Geometry: final body of the model. Coordinates: model frame, mm. A direction names the side the tool comes from. Give positions to 0.01 mm unless a question says otherwise; leave off trailing zeros. Write each loop counter-clockwise with the first axis right and the second up, starting at its lowest first coordinate (ties: lowest second). Pieces come first, ordered by that corner, then holes. Notation, with made-up numbers: (-5, 87) - (7, 87) arc R19 ccw to (7, 108) - close; hole circle Ø1 at (-20.75, -19). An arc over 180 degrees is marked (long way). One line per question, with ' | ' between items. Start each with the question number.
```python
from build123d import *

# Parameters (mm, degrees)
SKETCH_1_W               = 75
SKETCH_1_H               = 75
EXTRUDE_1_DEPTH          = 5.5
FILLET_1_R               = 5
SKETCH_2_R               = 3.5
CUT_EXTRUDE_1_DEPTH      = 54.31744555
PATTERN_CIRCULAR_1_COUNT = 4
SKETCH_3_R               = 10
CUT_EXTRUDE_2_DEPTH      = 3
SKETCH_4_R               = 35
EXTRUDE_2_DEPTH          = 7
SKETCH_5_R               = 30
EXTRUDE_3_DEPTH          = 55
SKETCH_6_W               = 50
SKETCH_6_H               = 55
EXTRUDE_4_DEPTH          = 26.5
FILLET_2_R               = 15
SKETCH_7_W               = 38
SKETCH_7_H               = 30
CUT_EXTRUDE_3_DEPTH      = 114.606777967
SKETCH_9_R               = 25
EXTRUDE_5_DEPTH          = 12.5
EXTRUDE_6_REACH          = 118.916
SKETCH_8_R               = 2.5
FILLET_3_R               = 15


with BuildPart() as part:
    # Sketch 1 → Extrude 1 (new body)
    with BuildSketch(Plane.XY):
        Rectangle(SKETCH_1_W, SKETCH_1_H)
    extrude(amount=EXTRUDE_1_DEPTH)

    # Fillet 1
    fillet_1_edges = [part.edges().sort_by_distance(p)[0] for p in [
        (-37.5, 37.5, 2.75),
        (37.5, 37.5, 2.75),
        (37.5, -37.5, 2.75),
        (-37.5, -37.5, 2.75),
    ]]
    fillet(fillet_1_edges, radius=FILLET_1_R)

    # Sketch 2 → Cut-Extrude 1 (cut, through all)
    with BuildSketch(Plane.XY.offset(5.5)):
        with Locations((-29, 29)):
            Circle(SKETCH_2_R)
    cut_extrude_1 = extrude(amount=-CUT_EXTRUDE_1_DEPTH, mode=Mode.SUBTRACT)

    # Pattern Circular 1: Cut-Extrude 1 ×4 about axis
    pattern_circular_1_axis = Axis((0, 0, 0), (0, 0, 1))
    for i in range(1, PATTERN_CIRCULAR_1_COUNT):
        add(cut_extrude_1.rotate(pattern_circular_1_axis, i * 360 / PATTERN_CIRCULAR_1_COUNT), mode=Mode.SUBTRACT)

    # Sketch 3 → Cut-Extrude 2 (cut)
    with BuildSketch(Plane.XY.offset(5.5)):
        Circle(SKETCH_3_R)
    extrude(amount=-CUT_EXTRUDE_2_DEPTH, mode=Mode.SUBTRACT)

    # Sketch 4 → Extrude 2 (add)
    with BuildSketch(Plane(origin=(0, 0, 0), x_dir=(-1, 0, 0), z_dir=(0, 0, -1))):
        with Locations(Location((0, 0, 0), (0, 0, 180))):
            Circle(SKETCH_4_R)
    extrude(amount=EXTRUDE_2_DEPTH)

    # Sketch 5 → Extrude 3 (add)
    with BuildSketch(Plane(origin=(0, 0, -7), x_dir=(-1, 0, 0), z_dir=(0, 0, -1))):
        Circle(SKETCH_5_R)
    extrude(amount=EXTRUDE_3_DEPTH)

    # Sketch 6 → Extrude 4 (add, symmetric)
    with BuildSketch(Plane(origin=(0, 0, 0), x_dir=(1, 0, 0), z_dir=(0, 1, 0))):
        with Locations((25, 34.5)):
            Rectangle(SKETCH_6_W, SKETCH_6_H)
    extrude(amount=EXTRUDE_4_DEPTH, both=True)

    # Fillet 2
    fillet_2_edges = [part.edges().sort_by_distance(p)[0] for p in [
        (50, 0, -7),
    ]]
    fillet(fillet_2_edges, radius=FILLET_2_R - 0.0001)  # a hair under: the kernel refuses the full size

    # Sketch 7 → Cut-Extrude 3 (cut, through all)
    with BuildSketch(Plane(origin=(50, 0, 0), x_dir=(0, 0, -1), z_dir=(1, 0, 0))):
        with Locations((43, 0)):
            Rectangle(SKETCH_7_W, SKETCH_7_H)
    extrude(amount=-CUT_EXTRUDE_3_DEPTH, mode=Mode.SUBTRACT)

    # Extrude 6: up to this face of the body (flat: up to its plane)
    extrude_6_end = Plane(part.part.faces().sort_by_distance((31.665133936, -26.5, -35.104709871))[0])
    # Sketch 8 → Extrude 6 (add, up to the picked face)
    with BuildSketch(Plane(origin=(0, 26.5, 0), x_dir=(1, 0, 0), z_dir=(0, 1, 0)), mode=Mode.PRIVATE) as extrude_6_sk1:
        with Locations(Location((36, 51.5, 0), (0, 0, 270))):
            Circle(SKETCH_8_R)
    extrude_6_tool1 = split(extrude(extrude_6_sk1.sketch, amount=-EXTRUDE_6_REACH, mode=Mode.PRIVATE), bisect_by=extrude_6_end, keep=Keep.BOTH, mode=Mode.PRIVATE)


with BuildPart() as body_2:
    # Sketch 9 → Extrude 5 (new, symmetric)
    with BuildSketch(Plane(origin=(0, 0, 0), x_dir=(1, 0, 0), z_dir=(0, 1, 0))):
        with Locations(Location((36, 51.5, 0), (0, 0, 270))):
            Circle(SKETCH_9_R)
    extrude(amount=EXTRUDE_5_DEPTH, both=True)


with BuildPart() as part_1:
    add(part.part)

    add(body_2.part)  # Extrude 6 merges body 2
    add(extrude_6_tool1.solids().sort_by(Axis((36, 26.5, -51.5), (0, -1, 0)))[0])

    # Fillet 3
    fillet_3_edges = [part_1.edges().sort_by_distance(p)[0] for p in [
        (50, 20.75, -62),
        (50, -20.75, -62),
    ]]
    fillet(fillet_3_edges, radius=FILLET_3_R)


solid = part_1.part
```
1) Section D-D, the plane x = 29. Output: boundary loops of the cut face in (y, z).
2) First-contact query: pin 1 Ø1.5 at (y, z) = (-12.5, -8.5) entering from +X; pin 2 Ø20 at (y, z) = (5.5, -30) entering from +X; pin 3 Ø4 at (y, z) = (-17, -4.5) entering from +X; pin 4 Ø11 at (x, y) = (-29, -29) entering from +Z. Flat tips, straight axial feed; report the tip coordinate or a pass-through.
3) Pull-direction query (Y, two-part tool) for faces 6 (the cylindrical face through (-36.07, -36, 2.79)), 7 (the cylindrical face through (-32.47, -29.46, 2.79)), 8 (the flat face through (-37.5, 0, 3)), 9 (the flat face through (0, 0, 2.5)); classes: +Y half, -Y half, draft (parallel to the pull), parting line (faces both ways), or undercut.
4) Reachability of faces 1 (the flat face through (37.5, 0, 3)), 2 (the cylindrical face through (45.72, -20.83, -57.49)), 3 (the cylindrical face through (27.12, -31.95, 2.79)), 4 (the cylindrical face through (45.72, 20.67, -57.49)), 5 (the flat face through (-31, 17, 0)) from +Z, -Z, +X, -X, +Y, -Y: full face, straight path, thin tool, end or side. Return the list, or none.
5) Section B-B, the plane x = 45. Output: boundary loops of the cut face in (y, z).
6) Line query: L1, parallel to X at y = -29, z = 1.3; L2, parallel to Y at x = 49, z = -35.5. Output: solid intervals per line, ascending.
7) Section C-C, the plane z = -51.5. Output: boundary loops of the cut face in (x, y), plus the area to 3 significant figures.
Answer key:
1) outline: (-37.5, 0) - (-32.5, 0) - (-32.5, 5.5) - (-37.5, 5.5) - close; (-26.5, -62) - (-15, -62) - (-15, -24) - (15, -24) - (15, -62) - (26.5, -62) - (26.5, -7) - (19.6, -7) - (19.6, 0) - (25.5, 0) - (25.5, 5.5) - (-25.5, 5.5) - (-25.5, 0) - (-19.6, 0) - (-19.6, -7) - (-26.5, -7) - close; (-12.5, -75.5) - (12.5, -75.5) - (12.5, -27.5) - (-12.5, -27.5) - close; (32.5, 0) - (37.5, 0) - (37.5, 5.5) - (32.5, 5.5) - close
2) pin 1: x = 42.9 | pin 2: x = 58.2 | pin 3: x = 31.62 | pin 4: z = 5.5
3) face 6: -Y half | face 7: undercut | face 8: draft | face 9: undercut
4) face 1: +Z, +X, +Y, -Y | face 2: -Z, +X, -Y | face 3: +Z | face 4: -Z, +X, +Y | face 5: none
5) outline: (-26.5, -58.18) - (-15, -58.18) - (-15, -24) - (15, -24) - (15, -58.18) - (26.5, -58.18) - (26.5, -10.82) - (-26.5, -10.82) - close; (-12.5, -74.82) - (12.5, -74.82) - (12.5, -28.18) - (-12.5, -28.18) - close
6) L1: -37.5 to -32.5, -25.5 to 25.5, 32.5 to 37.5 | L2: -26.5 to -15, -12.5 to 12.5, 15 to 26.5
7) outline: (-25.98, -15) arc R30 ccw to (14.06, -26.5) - (49.31, -26.5) - (49.31, -15) - (38.5, -15) - (38.5, -12.5) - (61, -12.5) - (61, 12.5) - (38.5, 12.5) - (38.5, 15) - (49.31, 15) - (49.31, 26.5) - (14.06, 26.5) arc R30 ccw to (-25.98, 15) - (33.5, 15) - (33.5, 12.5) - (11, 12.5) - (11, -12.5) - (33.5, -12.5) - (33.5, -15) - close | area: 3,030 mm^2
